```python
from build123d import *

# Parameters (mm, degrees)
SKETCH1_W           = 317.959323002
SKETCH1_H           = 237.284389444
BOSS_EXTRUDE1_DEPTH = 25.4
CUT_EXTRUDE1_START  = 25.4
SKETCH1_3_R         = 1.75
CUT_EXTRUDE1_DEPTH  = 6.35
SKETCH5_R           = 9.525
CUT_EXTRUDE2_DEPTH  = 26.4
CUT_EXTRUDE3_REACH  = 239.284
SKETCH6_W           = 11.775930683
SKETCH6_H           = 25.4
SKETCH6_W_2         = 11.132113684


with BuildPart() as part:
    # Sketch1 → Boss-Extrude1 (new body)
    with BuildSketch(Plane(origin=(0, 0, 0), x_dir=(1, 0, 0), z_dir=(0, 1, 0))):
        with Locations((114.5, 0)):
            Rectangle(SKETCH1_W, SKETCH1_H)
    extrude(amount=BOSS_EXTRUDE1_DEPTH)

    # Sketch1<3> → Cut-Extrude1 (cut)
    with BuildSketch(Plane(origin=(0, 0, 0), x_dir=(1, 0, 0), z_dir=(0, 1, 0)).offset(CUT_EXTRUDE1_START)):
        with Locations((24.5, 85.442194722)):
            Circle(SKETCH1_3_R)
        with Locations((84.5, 85.442194722)):
            Circle(SKETCH1_3_R)
        with Locations((144.5, 85.442194722)):
            Circle(SKETCH1_3_R)
        with Locations((204.5, 85.442194722)):
            Circle(SKETCH1_3_R)
        with Locations((24.5, -85.442194722)):
            Circle(SKETCH1_3_R)
        with Locations((84.5, -85.442194722)):
            Circle(SKETCH1_3_R)
        with Locations((144.5, -85.442194722)):
            Circle(SKETCH1_3_R)
        with Locations((204.5, -85.442194722)):
            Circle(SKETCH1_3_R)
    extrude(amount=-CUT_EXTRUDE1_DEPTH, mode=Mode.SUBTRACT)

    # Sketch5 → Cut-Extrude2 (cut, through all)
    with BuildSketch(Plane(origin=(0, 25.4, 0), x_dir=(1, 0, 0), z_dir=(0, 1, 0))):
        with Locations((-22.254661501, -93.242194722)):
            Circle(SKETCH5_R)
        with Locations((251.254661501, -93.242194722)):
            Circle(SKETCH5_R)
        with Locations((251.254661501, 93.337805278)):
            Circle(SKETCH5_R)
        with Locations((-22.254661501, 93.337805278)):
            Circle(SKETCH5_R)
    extrude(amount=-CUT_EXTRUDE2_DEPTH, mode=Mode.SUBTRACT)

    # Sketch6 → Cut-Extrude3 (cut, up to next)
    with BuildSketch(Plane.XY.offset(118.642194722), mode=Mode.PRIVATE) as cut_extrude3_sk1:
        with Locations((-43.787965342, 12.7)):
            Rectangle(SKETCH6_W, SKETCH6_H)
    cut_extrude3_tool1 = extrude(cut_extrude3_sk1.sketch, amount=-CUT_EXTRUDE3_REACH, mode=Mode.PRIVATE) & part.part
    add(cut_extrude3_tool1.solids().sort_by_distance((-43.787965, 12.7, 118.642195))[0], mode=Mode.SUBTRACT)
    # Sketch6 → Cut-Extrude3 (cut, up to next)
    with BuildSketch(Plane.XY.offset(118.642194722), mode=Mode.PRIVATE) as cut_extrude3_sk2:
        with Locations((272.466056842, 12.7)):
            Rectangle(SKETCH6_W_2, SKETCH6_H)
    cut_extrude3_tool2 = extrude(cut_extrude3_sk2.sketch, amount=-CUT_EXTRUDE3_REACH, mode=Mode.PRIVATE) & part.part
    add(cut_extrude3_tool2.solids().sort_by_distance((272.466057, 12.7, 118.642195))[0], mode=Mode.SUBTRACT)


solid = part.part
```
Verification items for the finished model (mm, model axes). Coordinates: 2 decimals unless noted, no trailing zeros. Loops run counter-clockwise (first coordinate to the right, second up) from the corner with the lowest first, then second, coordinate; pieces in that order, holes last. Notation, with made-up numbers: (-18.5, 76.5) -> (11.5, 76.5) arc R19 cw to (11.5, 104.5) -> close; hole circle Ø2 at (22, 13.25). An arc over 180 degrees is marked (long way). Answer in a Markdown table with one row per item.
1) Draft check along Z on faces 1 (the face through (243.696, 12.878, -87.542)), 2 (the face through (112, 0, -2)), 3 (the face through (112, 13, 118.642)). Enter one of: released by +Z, released by -Z, zero draft, split by the parting line, or undercut.
The answers:
| item | result |
|---|---|
| face 1 | undercut |
| face 2 | zero draft |
| face 3 | released by +Z |
2) Section check A-A (y = 11.25). Record the cut outline in (x, z) (3 decimals), and give its area (3 significant figures).
The answers:
| item | result |
|---|---|
| outline | (-37.9, -118.642) -> (266.9, -118.642) -> (266.9, 118.642) -> (-37.9, 118.642) -> close; hole circle Ø19.05 at (-22.255, -93.338); hole circle Ø19.05 at (-22.255, 93.242); hole circle Ø19.05 at (251.255, -93.338); hole circle Ø19.05 at (251.255, 93.242) |
| area | 71,200 mm2 |
3) Depth check by flat-ended pin: P1, Ø1, axis at x = 25, z = -85.5, coming from the +Y side. Enter the tip coordinate at first touch or a pass-through.
The answers:
| item | result |
|---|---|
| P1 | stops at y = 19.05 |
4) Scan lines: line 1 along Z through (x, y) = (24.5, 21.5); line 2 along X through (y, z) = (21, -96); line 3 along Z through (x, y) = (252.5, 16). Record each from-to range of solid material in increasing order. Write a range as from..to.
The answers:
| item | result |
|---|---|
| line 1 | z = -118.64..-87.19, -83.69..83.69, 87.19..118.64 |
| line 2 | x = -37.9..-31.4, -13.11..242.11, 260.4..266.9 |
| line 3 | z = -118.64..-102.78, -83.89..83.8, 102.69..118.64 |
